from build123d import *

# Parameters (mm, degrees)
REVOLVE1_ANGLE      = 57
BOSS_EXTRUDE1_DEPTH = 25.4
SKETCH8_R           = 152.4
CUT_EXTRUDE3_DEPTH  = 257.048
SKETCH13_W          = 16.387620484
SKETCH13_H          = 127
CUT_EXTRUDE5_DEPTH  = 1.778


with BuildPart() as part:
    # Sketch1 → Revolve1 (revolve)
    with BuildSketch(Plane.XY):
        with BuildLine():
            Line((-59.991213716, 144.035687339), (-8.193810242, 180.296949153))
            ThreePointArc((-8.193810242, 180.296949153), (0, 182.88), (8.193810242, 180.296949153))
            Line((8.193810242, 180.296949153), (59.991213716, 144.035687339))
            add(Edge.make_bspline(
                [(59.991213716, 144.035687339), (62.78248672, 142.0840471), (62.441206007, 139.021062406)],
                knots=[0, 0, 0, 1, 1, 1], degree=2))
            ThreePointArc((62.441206007, 139.021062406), (0, 152.4), (-62.441206007, 139.021062406))
            add(Edge.make_bspline(
                [(-59.991213716, 144.035687339), (-62.78248672, 142.0840471), (-62.441206007, 139.021062406)],
                knots=[0, 0, 0, 1, 1, 1], degree=2))
        make_face()
    revolve(axis=Axis((0, 0, 0), (-1, 0, 0)), revolution_arc=REVOLVE1_ANGLE)

    # Sketch3 → Boss-Extrude1 (add)
    with BuildSketch(Plane.XY):
        with BuildLine():
            Line((-59.991213716, 144.035687339), (-8.193810242, 180.296949153))
            ThreePointArc((-8.193810242, 180.296949153), (0, 182.88), (8.193810242, 180.296949153))
            Line((8.193810242, 180.296949153), (59.991213716, 144.035687339))
            add(Edge.make_bspline(
                [(59.991213716, 144.035687339), (62.78248672, 142.0840471), (62.441206007, 139.021062406)],
                knots=[0, 0, 0, 1, 1, 1], degree=2))
            ThreePointArc((62.441206007, 139.021062406), (0, 152.4), (-62.441206007, 139.021062406))
            add(Edge.make_bspline(
                [(-59.991213716, 144.035687339), (-62.78248672, 142.0840471), (-62.441206007, 139.021062406)],
                knots=[0, 0, 0, 1, 1, 1], degree=2))
        make_face()
    extrude(amount=BOSS_EXTRUDE1_DEPTH)

    # Sketch7 → Cut-Revolve2 (revolve, cut)
    with BuildSketch(Plane.XY.offset(12.7)):
        Polygon((-18.85509192, 148.029004366), (-21.456080621, 146.208157646), (-33.109499632, 162.854485329), (-27.584999632, 166.721963764), (-28.163260355, 161.325258604), align=None)
    cut_revolve2 = revolve(axis=Axis((-21.456080621, 146.208157646, 12.7), (-0.57349503, 0.81920904, 0)), mode=Mode.SUBTRACT)

    # Mirror2: Cut-Revolve2 across plane
    add(cut_revolve2.mirror(Plane(origin=(0, 0, 0), x_dir=(0, 0, 1), z_dir=(1, 0, 0))), mode=Mode.SUBTRACT)

    # Sketch8 → Cut-Extrude3 (cut)
    with BuildSketch(Plane.XY.offset(25.4)):
        Circle(SKETCH8_R)
    extrude(amount=-CUT_EXTRUDE3_DEPTH, mode=Mode.SUBTRACT)

    # Sketch13 → Cut-Extrude5 (cut)
    with BuildSketch(Plane(origin=(0, 167.069193294, -74.383997286), x_dir=(1, 0, 0), z_dir=(0, 0.913545458, -0.406736643))):
        Rectangle(SKETCH13_W, SKETCH13_H)
    extrude(amount=-CUT_EXTRUDE5_DEPTH, mode=Mode.SUBTRACT)

    # Sketch14 → Cut-Revolve4 (revolve, cut)
    with BuildSketch(Plane(origin=(0, 0, 0), x_dir=(0, 0, -1), z_dir=(1, 0, 0))):
        Polygon((73.660819534, 165.44490947), (67.500143032, 168.18781937), (69.097003878, 163.000445517), (60.429201972, 143.532243688), (63.3297088, 142.240854846), align=None)
    revolve(axis=Axis((0, 165.44490947, -73.660819534), (0, -0.913545458, 0.406736643)), mode=Mode.SUBTRACT)


solid = part.part
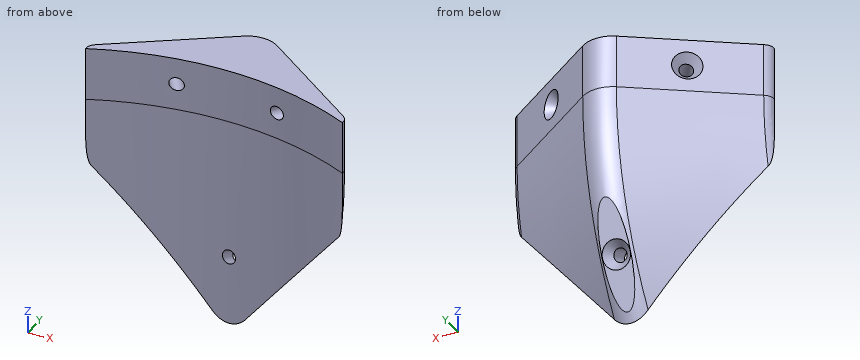
Design review of the part built by this model. Coordinates are the model's own, in mm. Coordinates: 2 decimals unless noted, no trailing zeros. Order: outer loops, then holes, each group sorted by start corner. A loop starts at its lowest first (then second) coordinate and runs counter-clockwise, first axis right, second up. Notation, with made-up numbers: M 18,77.5 L 47,77.5 A32 cw 47,111.5 Z; hole C 2.5,19.5 d5. An arc over 180 degrees is marked long. Use a Markdown table: item, result.
(1) Add section A-A (x = -41). Give the boundary of the cut face in (y, z), then the cut area to 3 significant figures.
Worked answers:
| item | result |
|---|---|
| outline | M 146.78,-56.64 A157.33 ccw 157.33,0 L 157.33,25.4 L 146.78,25.4 Z |
| area | 669 mm2 |
(2) Add section B-B (x = 16). Give the boundary of the cut face in (y, z), then the cut area to 3 significant figures.
Worked answers:
| item | result |
|---|---|
| outline | M 151.56,-87.16 A174.83 ccw 174.83,0 L 174.83,25.4 L 151.56,25.4 Z |
| area | 1,960 mm2 |
(3) Wall thickness on probe 1 along Y at (x, z) = (-25.5, -49); probe 2 along X at (y, z) = (158, -16); probe 3 along Y at (x, z) = (28.5, 0): over which ranges is each line inside the solid? List them lowest first.
Worked answers:
| item | result |
|---|---|
| probe 1 | y = 150.25 to 160.89 |
| probe 2 | x = -38.89 to 38.89 |
| probe 3 | y = 149.71 to 166.08 |
(4) For P1, Ø6, axis at x = 17.5, z = -23, coming from the -Y side; P2, Ø1.5, axis at x = 18, z = -34, coming from the -Y side; P3, Ø1, axis at y = 148.5, z = 6, coming from the -X side, all flat-tipped, find the tip position at first contact; note any pin that passes through.
Worked answers:
| item | result |
|---|---|
| P1 | stops at y = 151.01 |
| P2 | stops at y = 151.24 |
| P3 | stops at x = -54.33 |
